The listing builds one solid part. Answer for the finished solid, in the listing's coordinates (mm). A direction names the side the tool comes from. Give positions to 0.01 mm unless a question says otherwise; leave off trailing zeros. Write each loop counter-clockwise with the first axis right and the second up, starting at its lowest first coordinate (ties: lowest second). Pieces come first, ordered by that corner, then holes. Notation, with made-up numbers: (41, 29) - (92, 29) arc R32 cw to (92, 66) - close; hole circle Ø10 at (3.5, 8). An arc over 180 degrees is marked (long way). Answer in a Markdown table with one row per item. Add a question column.
from build123d import *

# Parameters (mm, degrees)
SKETCH1_W           = 501
SKETCH1_H           = 511
BOSS_EXTRUDE1_DEPTH = 0.8
SKETCH2_W           = 501
SKETCH2_H           = 1.003667413
BOSS_EXTRUDE2_DEPTH = 32
SKETCH3_W           = 1
SKETCH3_H           = 509.996332587
BOSS_EXTRUDE3_DEPTH = 32
SKETCH7_W           = 1
SKETCH7_H           = 509.996332587
BOSS_EXTRUDE4_DEPTH = 34
SKETCH8_W           = 499
SKETCH8_H           = 1
BOSS_EXTRUDE5_DEPTH = 32


with BuildPart() as part:
    # Sketch1 → Boss-Extrude1 (new body)
    with BuildSketch(Plane.XY):
        with Locations((250.5, 255.5)):
            Rectangle(SKETCH1_W, SKETCH1_H)
    extrude(amount=BOSS_EXTRUDE1_DEPTH)

    # Sketch2 → Boss-Extrude2 (add)
    with BuildSketch(Plane.XY.offset(0.8)):
        with Locations((250.5, 510.498166294)):
            Rectangle(SKETCH2_W, SKETCH2_H)
    extrude(amount=BOSS_EXTRUDE2_DEPTH)

    # Sketch3 → Boss-Extrude3 (add)
    with BuildSketch(Plane.XY.offset(0.8)):
        with Locations((500.5, 254.998166294)):
            Rectangle(SKETCH3_W, SKETCH3_H)
    extrude(amount=BOSS_EXTRUDE3_DEPTH)

    # Sketch7 → Boss-Extrude4 (add)
    with BuildSketch(Plane(origin=(0, 0, 0), x_dir=(-1, 0, 0), z_dir=(0, 0, -1))):
        with Locations((-0.5, 254.998166294)):
            Rectangle(SKETCH7_W, SKETCH7_H)
    extrude(amount=-BOSS_EXTRUDE4_DEPTH)

    # Sketch8 → Boss-Extrude5 (add)
    with BuildSketch(Plane.XY.offset(0.8)):
        with Locations((250.5, 0.5)):
            Rectangle(SKETCH8_W, SKETCH8_H)
    extrude(amount=BOSS_EXTRUDE5_DEPTH)


solid = part.part
1. Given pin 1 Ø2 at (x, y) = (436, 222) entering from -Z; pin 2 Ø0.5 at (x, z) = (0.5, 33.5) entering from +Y; pin 3 Ø2 at (x, y) = (413, 395) entering from +Z, each flat-ended and moving along its own axis, determine where each tip first touches the part or whether it passes through.
2. The mould has two halves that part along Y. Classify faces 1 (the face through (247, 511, 16)), 2 (the face through (500, 252, 17)), 3 (the face through (247, 0, 17)): +Y half, -Y half, draft (parallel to the pull), parting line (faces both ways), or undercut.
3. A tool of negligible diameter and unlimited length cuts with its end or side. For faces 4 (the face through (0, 252, 17)), 5 (the face through (247, 1, 17)), from which of +Z, -Z, +X, -X, +Y, -Y can it reach the whole face along a straight path? Write none if from no direction.
4. Section C-C (y = 259) is taken. Give the vertices of the cut face in (x, z), and give its area (3 significant figures).
5. Section B-B (x = 367) is taken. Give the vertices of the cut face in (y, z), and give its area (3 significant figures).
6. Straight lines are drawn through the part: L1, parallel to X at y = 93.5, z = 31.5; L2, parallel to Y at x = 331, z = 6; L3, parallel to Z at x = 357.5, y = 184.5. For each, find the intervals that lie inside material, in ascending order. Write a range as [from, to].
7. Section A-A (z = 23) is taken. Give the vertices of the cut face in (x, y).
Geometry check:
| question | item | result |
|---|---|---|
| 1 | pin 1 | z = 0 |
| 1 | pin 2 | y = 510 |
| 1 | pin 3 | z = 0.8 |
| 2 | face 1 | +Y half |
| 2 | face 2 | undercut |
| 2 | face 3 | -Y half |
| 3 | face 4 | +Z, -Z, -X, +Y, -Y |
| 3 | face 5 | +Z |
| 4 | outline | (0, 0) - (501, 0) - (501, 32.8) - (500, 32.8) - (500, 0.8) - (1, 0.8) - (1, 34) - (0, 34) - close |
| 4 | area | 466 mm² |
| 5 | outline | (0, 0) - (511, 0) - (511, 32.8) - (510, 32.8) - (510, 0.8) - (1, 0.8) - (1, 32.8) - (0, 32.8) - close |
| 5 | area | 473 mm² |
| 6 | L1 | [0, 1], [500, 501] |
| 6 | L2 | [0, 1], [510, 511] |
| 6 | L3 | [0, 0.8] |
| 7 | outline | (0, 0) - (501, 0) - (501, 511) - (0, 511) - close; hole (1, 1) - (500, 1) - (500, 510) - (1, 510) - close |
